Geometry: see drawing. Coordinates: mm, zero at the bounding-box minimum. Round coordinates to 2 decimals unless told otherwise and drop trailing zeros. Write each loop counter-clockwise with the first axis right and the second up, starting at its lowest first coordinate (ties: lowest second). Pieces come first, ordered by that corner, then holes. Notation, with made-up numbers: M 83,33 L 138,33 A21 ccw 138,68 Z; hole C 47.25,2 d5. An arc over 180 degrees is marked long. Use one line per item in the form item = value. Start each with the question number.
Item 1: Section query B-B (y = 8). Return loops of the section in (x, z), and give its area (3 significant figures).
Item 2: Ray query, probe 1 along X at (y, z) = (8.25, 5.75); probe 2 along X at (y, z) = (8, 18). Return the intervals inside material, ascending.
Item 3: Section query A-A (z = 5). Return loops of the section in (x, y), and give its area (3 significant figures).
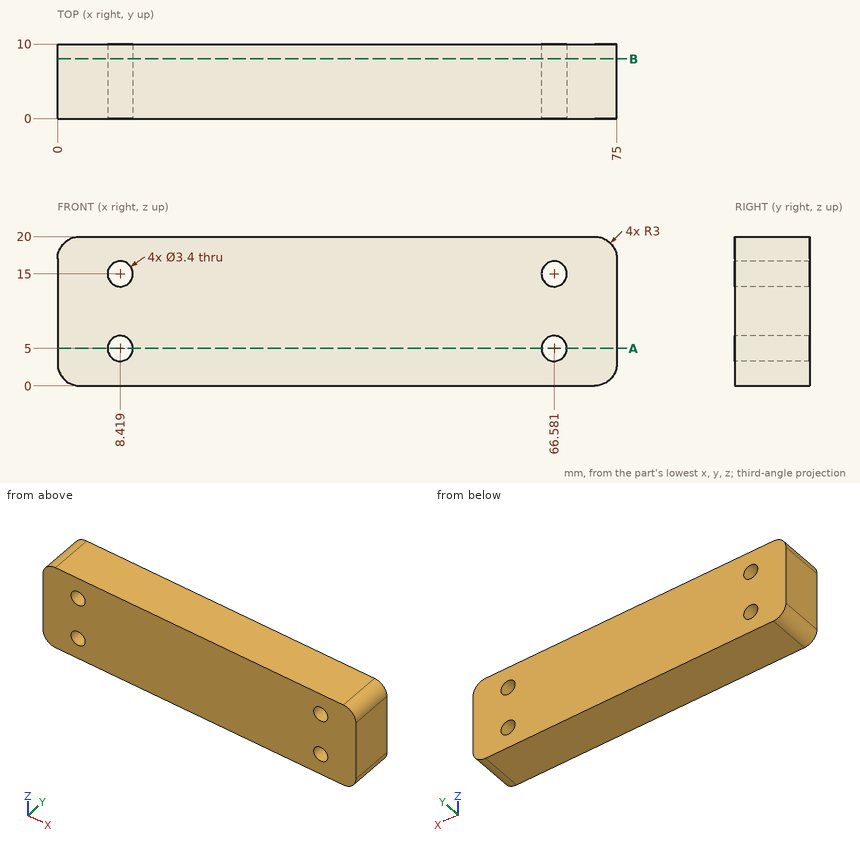
Working result:
q1.outline = M 0,3 A3 ccw 3,0 L 72,0 A3 ccw 75,3 L 75,17 A3 ccw 72,20 L 3,20 A3 ccw 0,17 Z; hole C 8.42,5 d3.4; hole C 8.42,15 d3.4; hole C 66.58,5 d3.4; hole C 66.58,15 d3.4
q1.area = 1,460 mm²
q2.probe_1 = 0 to 6.89, 9.94 to 65.06, 68.11 to 75
q2.probe_2 = 0.17 to 74.83
q3.outline = M 0,0 L 6.72,0 L 6.72,10 L 0,10 Z; M 10.12,0 L 64.88,0 L 64.88,10 L 10.12,10 Z; M 68.28,0 L 75,0 L 75,10 L 68.28,10 Z
q3.area = 682 mm²
